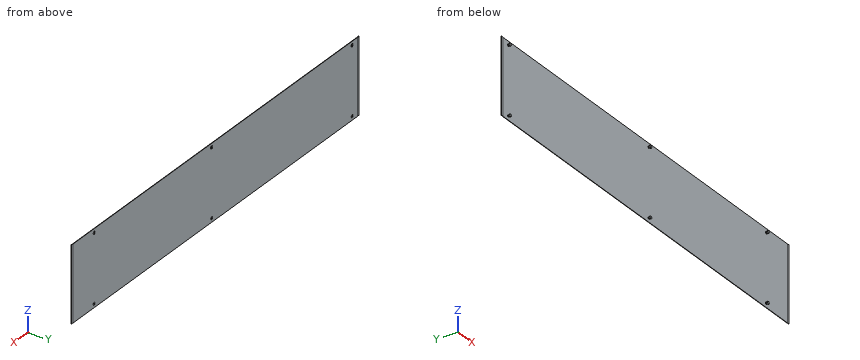
```python
from build123d import *

# Parameters (mm, degrees)
BOSS_EXTRUDE1_DEPTH    = 86.5
CUT_EXTRUDE1_DEPTH     = 1.2
BOSS_EXTRUDE2_DEPTH    = 2.4
LPATTERN1_COUNT        = 2
LPATTERN1_PITCH        = 871
LPATTERN1_COPY_3_DEPTH = 1.2
LPATTERN1_COPY_4_DEPTH = 2.4
LPATTERN2_COUNT        = 2
LPATTERN2_PITCH        = 474.5
LPATTERN2_COPY_3_DEPTH = 1.2
LPATTERN2_COPY_4_DEPTH = 2.4


with BuildPart() as part:
    # Sketch1 → Boss-Extrude1 (new, symmetric)
    with BuildSketch(Plane.XY):
        Polygon((15.3, 14.615402534), (15.369756474, 13.617838484), (20.834920769, 14), (981.005079231, 14), (986.270243526, 13.631823846), (986.34, 14.629387897), (981.04, 15), (20.8, 15), align=None)
    extrude(amount=BOSS_EXTRUDE1_DEPTH, both=True)

    # Sketch3 → Cut-Revolve1 (revolve, cut)
    with BuildSketch(Plane.XY.offset(77.5)):
        Polygon((39, 15), (42.5, 15), (41.5, 14), (39, 14), align=None)
    cut_revolve1 = revolve(axis=Axis((39, 14, 77.5), (0, 1, 0)), mode=Mode.SUBTRACT)

    # Sketch4 → Revolve1 (revolve)
    with BuildSketch(Plane.XY.offset(77.5), mode=Mode.PRIVATE) as revolve1_sk:
        Polygon((39, 14.8), (42, 14.8), (42, 14.5), (40.5, 13), (40.5, 9.3), (39, 9.3), align=None)
    revolve1 = revolve(revolve1_sk.sketch.rotate(Axis((39, 15, 77.5), (0, -1, 0)), 90), axis=Axis((39, 15, 77.5), (0, -1, 0)))

    # Sketch5 → Cut-Extrude1 (cut)
    with BuildSketch(Plane(origin=(0, 14.8, 0), x_dir=(1, 0, 0), z_dir=(0, 1, 0))):
        Polygon((39, -76.345299462), (38, -76.922649731), (38, -78.077350269), (39, -78.654700538), (40, -78.077350269), (40, -76.922649731), align=None)
    cut_extrude1 = extrude(amount=-CUT_EXTRUDE1_DEPTH, mode=Mode.SUBTRACT)

    # Sketch6 → Boss-Extrude2 (add)
    with BuildSketch(Plane(origin=(0, 11.4, 0), x_dir=(1, 0, 0), z_dir=(0, 1, 0))):
        Polygon((35.824573519, -77.5), (37.41228676, -80.25), (40.58771324, -80.25), (42.175426481, -77.5), (40.58771324, -74.75), (37.41228676, -74.75), align=None)
    boss_extrude2 = extrude(amount=-BOSS_EXTRUDE2_DEPTH)

    # Mirror1: Cut-Revolve1, Revolve1, Cut-Extrude1, Boss-Extrude2 across plane
    add(cut_revolve1.mirror(Plane.XY), mode=Mode.SUBTRACT)
    add(revolve1.mirror(Plane.XY))
    add(cut_extrude1.mirror(Plane.XY), mode=Mode.SUBTRACT)
    add(boss_extrude2.mirror(Plane.XY))

    # LPattern1: Cut-Revolve1, Revolve1, Cut-Extrude1, Boss-Extrude2 ×2
    with Locations(*[(i * LPATTERN1_PITCH, 0, 0) for i in range(1, LPATTERN1_COUNT)]):
        add(cut_revolve1, mode=Mode.SUBTRACT)
        add(revolve1)
        add(cut_extrude1, mode=Mode.SUBTRACT)
        add(boss_extrude2)

    # LPattern1 copy 1 sketch → LPattern1 copy 1 (revolve, cut)
    with BuildSketch(Plane(origin=(871, 0, -77.5), x_dir=(1, 0, 0), z_dir=(0, 0, -1))):
        Polygon((39, -15), (42.5, -15), (41.5, -14), (39, -14), align=None)
    revolve(axis=Axis((910, 14, -77.5), (0, -1, 0)), mode=Mode.SUBTRACT)

    # LPattern1 copy 2 sketch → LPattern1 copy 2 (revolve)
    with BuildSketch(Plane(origin=(871, 0, -77.5), x_dir=(1, 0, 0), z_dir=(0, 0, -1))):
        Polygon((39, -14.8), (42, -14.8), (42, -14.5), (40.5, -13), (40.5, -9.3), (39, -9.3), align=None)
    revolve(axis=Axis((910, 15, -77.5), (0, 1, 0)))

    # LPattern1 copy 3 sketch → LPattern1 copy 3 (cut)
    with BuildSketch(Plane(origin=(871, 14.8, 0), x_dir=(1, 0, 0), z_dir=(0, 1, 0))):
        Polygon((39, 76.345299462), (38, 76.922649731), (38, 78.077350269), (39, 78.654700538), (40, 78.077350269), (40, 76.922649731), align=None)
    extrude(amount=-LPATTERN1_COPY_3_DEPTH, mode=Mode.SUBTRACT)

    # LPattern1 copy 4 sketch → LPattern1 copy 4 (add)
    with BuildSketch(Plane(origin=(871, 11.4, 0), x_dir=(1, 0, 0), z_dir=(0, 1, 0))):
        Polygon((35.824573519, 77.5), (37.41228676, 80.25), (40.58771324, 80.25), (42.175426481, 77.5), (40.58771324, 74.75), (37.41228676, 74.75), align=None)
    extrude(amount=-LPATTERN1_COPY_4_DEPTH)

    # LPattern2: Cut-Revolve1, Revolve1, Cut-Extrude1, Boss-Extrude2 ×2
    with Locations(*[(i * LPATTERN2_PITCH, 0, 0) for i in range(1, LPATTERN2_COUNT)]):
        add(cut_revolve1, mode=Mode.SUBTRACT)
        add(revolve1)
        add(cut_extrude1, mode=Mode.SUBTRACT)
        add(boss_extrude2)

    # LPattern2 copy 1 sketch → LPattern2 copy 1 (revolve, cut)
    with BuildSketch(Plane(origin=(474.5, 0, -77.5), x_dir=(1, 0, 0), z_dir=(0, 0, -1))):
        Polygon((39, -15), (42.5, -15), (41.5, -14), (39, -14), align=None)
    revolve(axis=Axis((513.5, 14, -77.5), (0, -1, 0)), mode=Mode.SUBTRACT)

    # LPattern2 copy 2 sketch → LPattern2 copy 2 (revolve)
    with BuildSketch(Plane(origin=(474.5, 0, -77.5), x_dir=(1, 0, 0), z_dir=(0, 0, -1))):
        Polygon((39, -14.8), (42, -14.8), (42, -14.5), (40.5, -13), (40.5, -9.3), (39, -9.3), align=None)
    revolve(axis=Axis((513.5, 15, -77.5), (0, 1, 0)))

    # LPattern2 copy 3 sketch → LPattern2 copy 3 (cut)
    with BuildSketch(Plane(origin=(474.5, 14.8, 0), x_dir=(1, 0, 0), z_dir=(0, 1, 0))):
        Polygon((39, 76.345299462), (38, 76.922649731), (38, 78.077350269), (39, 78.654700538), (40, 78.077350269), (40, 76.922649731), align=None)
    extrude(amount=-LPATTERN2_COPY_3_DEPTH, mode=Mode.SUBTRACT)

    # LPattern2 copy 4 sketch → LPattern2 copy 4 (add)
    with BuildSketch(Plane(origin=(474.5, 11.4, 0), x_dir=(1, 0, 0), z_dir=(0, 1, 0))):
        Polygon((35.824573519, 77.5), (37.41228676, 80.25), (40.58771324, 80.25), (42.175426481, 77.5), (40.58771324, 74.75), (37.41228676, 74.75), align=None)
    extrude(amount=-LPATTERN2_COPY_4_DEPTH)


solid = part.part
```
Could you check a few things on this model? Use its own coordinates, in mm. Round coordinates to 2 decimals unless told otherwise and drop trailing zeros. Write each loop counter-clockwise with the first axis right and the second up, starting at its lowest first coordinate (ties: lowest second). Pieces come first, ordered by that corner, then holes.
(1) If I drill on probe 1 along X at (y, z) = (10.6, 76); probe 2 along X at (y, z) = (12.5, -78.5); probe 3 along Y at (x, z) = (811.5, -14), over which ranges is the centre line in solid material (lowest first)?
Findings below:
probe 1: x = 36.69 to 41.31, 511.19 to 515.81, 907.69 to 912.31
probe 2: x = 37.88 to 40.12, 512.38 to 514.62, 908.88 to 911.12
probe 3: y = 14 to 15
(2) Suppose I cut it at A-A on y = 10.5. State how many separate pieces and enclosed holes the cut face has, and give its area (3 significant figures).
Findings below:
separate pieces: 6
enclosed holes: 0
area: 157 mm2
(3) Suppose I cut it at C-C on x = 735.5. Write out the boundary of the cut face in (y, z).
Findings below:
outline: (14, -86.5) - (15, -86.5) - (15, 86.5) - (14, 86.5) - close
(4) For pin 1 (0.7 mm diameter, centred on x = 39.5, y = 10, fed in from +Z); pin 2 (1.2 mm diameter, centred on x = 910, y = 10, fed in from -Z); pin 3 (1.8 mm diameter, centred on x = 908.5, z = 77, fed in from +Y); pin 4 (1.5 mm diameter, centred on y = 11.5, z = 8.5, fed in from -X), each with a flat end and sliding along its axis, tell me the tip position at first contact or that it passes through.
Findings below:
pin 1: stops at z = 80.25
pin 2: stops at z = -80.25
pin 3: stops at y = 14.8
pin 4: passes through
(5) Suppose I cut it at B-B on z = -46. Write out the boundary of the cut face in (x, y), and give its area (3 significant figures).
Findings below:
outline: (15.3, 14.62) - (15.37, 13.62) - (20.83, 14) - (981.01, 14) - (986.27, 13.63) - (986.34, 14.63) - (981.04, 15) - (20.8, 15) - close
area: 971 mm2
